Check sheet for the modelled part. Datum: model origin and axes. Units: mm. Face numbers are marked on the shaded views. Coordinates: 2 decimals unless noted, no trailing zeros. Loops run counter-clockwise (first coordinate to the right, second up) from the corner with the lowest first, then second, coordinate; pieces in that order, holes last. Notation, with made-up numbers: (47.25, 31) -> (100.25, 31) arc R27 cw to (100.25, 52) -> close; hole circle Ø9 at (23, -29.75). An arc over 180 degrees is marked (long way). Use one line per item in the form item = value.
from build123d import *

# Parameters (mm, degrees)
EXTRUDE_START       = -37
EXTRUDE_1_DEPTH     = 59
CUT_EXTRUDE_1_DEPTH = 58.416112721
SKETCH_5_R          = 4
EXTRUDE_2_DEPTH     = 15.1
SKETCH_6_R          = 4.8
EXTRUDE_3_DEPTH     = 1
FILLET_1_R          = 1.81
SKETCH_7_R          = 3.4
CUT_EXTRUDE_2_DEPTH = 54.005306338


with BuildPart() as part:
    # 草图3 → 凸台-拉伸1 (new body)
    with BuildSketch(Plane.XY.offset(EXTRUDE_START)):
        Polygon((-6.05, 3), (-6.05, 40), (-9.05, 40), (-9.05, 0), (9.05, 0), (9.05, 40), (6.05, 40), (6.05, 3), align=None)
    extrude(amount=EXTRUDE_1_DEPTH)

    # 草图4 → 切除-拉伸1 (cut, through all)
    with BuildSketch(Plane(origin=(9.05, 0, 0), x_dir=(0, 0, -1), z_dir=(1, 0, 0))):
        with BuildLine():
            Line((-7.5, 24.007504693), (-7.5, 3))
            Line((-7.5, 3), (-22, 3))
            Line((-22, 3), (-22, 40))
            Line((-22, 40), (37, 40))
            Line((37, 40), (37, 3))
            Line((37, 3), (26.673582437, 3))
            Line((26.673582437, 3), (8.313843876, 34.8))
            ThreePointArc((8.313843876, 34.8), (-5.411568553, 37.929371085), (-7.5, 24.007504693))
        make_face()
    extrude(amount=-CUT_EXTRUDE_1_DEPTH, mode=Mode.SUBTRACT)

    # 草图5 → 凸台-拉伸2 (add)
    with BuildSketch(Plane(origin=(9.05, 0, 0), x_dir=(0, 0, -1), z_dir=(1, 0, 0))):
        with Locations(Location((0, 30, 0), (0, 0, 90))):
            Circle(SKETCH_5_R)
    extrude(amount=-EXTRUDE_2_DEPTH)

    # 草图6 → 凸台-拉伸3 (add)
    with BuildSketch(Plane(origin=(9.05, 0, 0), x_dir=(0, 0, -1), z_dir=(1, 0, 0))):
        with Locations(Location((0, 30, 0), (0, 0, 270))):
            Circle(SKETCH_6_R)
    extrude_3 = extrude(amount=EXTRUDE_3_DEPTH)

    # 镜向1: 凸台-拉伸3 across plane
    add(extrude_3.mirror(Plane(origin=(0, 0, 0), x_dir=(0, 0, 1), z_dir=(1, 0, 0))))

    # 圆角1
    fillet_1_edges = [part.edges().sort_by_distance(p)[0] for p in [
        (9.05, 1.5, 22),
        (-9.05, 1.5, -37),
        (-9.05, 1.5, 22),
        (9.05, 1.5, -37),
    ]]
    fillet(fillet_1_edges, radius=FILLET_1_R)

    # 草图7 → 切除-拉伸2 (cut, through all)
    with BuildSketch(Plane(origin=(0, 3, 0), x_dir=(1, 0, 0), z_dir=(0, 1, 0))):
        with Locations(Location((0, -15, 0), (0, 0, 270))):
            Circle(SKETCH_7_R)
        with Locations(Location((0, 30, 0), (0, 0, 270))):
            Circle(SKETCH_7_R)
    extrude(amount=-CUT_EXTRUDE_2_DEPTH, mode=Mode.SUBTRACT)


solid = part.part
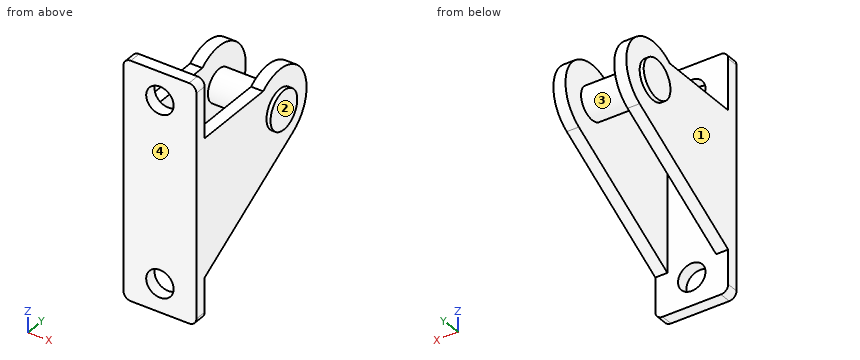
(1) Section check D-D, the plane y = 15.5. Record the boundary of the cut face in (x, z), plus the area to 3 significant figures.
Established:
outline = (-9.05, -19.46) -> (-6.05, -19.46) -> (-6.05, 7.5) -> (-9.05, 7.5) -> close; (6.05, -19.46) -> (9.05, -19.46) -> (9.05, 7.5) -> (6.05, 7.5) -> close
area = 162 mm²
(2) Scan lines: line 1 along X through (y, z) = (1.85, -30); line 2 along X through (y, z) = (33, -7); line 3 along Y through (x, z) = (-2, -8.5). Record each from-to range of solid material in increasing order.
Established:
line_1 = -9.05 to -3.4, 3.4 to 9.05
line_2 = -9.05 to -6.05, 6.05 to 9.05
line_3 = 0 to 3
(3) Section check B-B, the plane x = 0. Record the boundary of the cut face in (y, z).
Established:
outline = (0, -37) -> (3, -37) -> (3, -33.4) -> (0, -33.4) -> close; (0, -26.6) -> (3, -26.6) -> (3, 11.6) -> (0, 11.6) -> close; (0, 18.4) -> (3, 18.4) -> (3, 22) -> (0, 22) -> close; circle Ø8 at (30, 0)
(4) Section check C-C, the plane z = -30. Record the boundary of the cut face in (x, y), plus the area to 3 significant figures.
Established:
outline = (-9.05, 0) -> (-3.4, 0) -> (-3.4, 3) -> (-9.05, 3) -> close; (3.4, 0) -> (9.05, 0) -> (9.05, 3) -> (3.4, 3) -> close
area = 33.9 mm²
(5) Go/stop test with flat-tipped pins: P1, Ø1, axis at x = -3, y = 28, coming from the -Z side; P2, Ø3.5, axis at x = -8, y = 9, coming from the +Z side; P3, Ø6, axis at x = -2, z = -22, coming from the +Y side; P4, Ø10, axis at x = 6.5, z = -2.5, coming from the +Y side. Record where each tip stops, or that it passes through.
Established:
P1 = -3.71
P2 = 7.5
P3 = 3
P4 = 39.6
(6) Mould release check, pull along X, two halves, no side actions. Record for the marked faces 1, 2, 3 and 4: +X half, -X half, draft (parallel to the pull), parting line (faces both ways), or undercut.
Established:
face_1 = -X half
face_2 = +X half
face_3 = undercut
face_4 = draft
(7) Section check A-A, the plane z = 0. Record the boundary of the cut face in (x, y), plus the area to 3 significant figures.
Established:
outline = (-10.05, 25.2) -> (-9.05, 25.2) -> (-9.05, 0) -> (9.05, 0) -> (9.05, 25.2) -> (10.05, 25.2) -> (10.05, 34.8) -> (9.05, 34.8) -> (9.05, 39.6) -> (6.05, 39.6) -> (6.05, 34) -> (-6.05, 34) -> (-6.05, 39.6) -> (-9.05, 39.6) -> (-9.05, 34.8) -> (-10.05, 34.8) -> close; hole (-6.05, 3) -> (6.05, 3) -> (6.05, 26) -> (-6.05, 26) -> close
area = 390 mm²
